```python
from build123d import *

# Parameters (mm, degrees)
MODEL_R                 = 6
MODEL_W                 = 24
MODEL_H                 = 3
SALIENTE_EXTRUIR1_DEPTH = 3


with BuildPart() as part:
    # Model → Saliente-Extruir1 (new body)
    with BuildSketch(Plane.XY):
        Polygon((11.392528896, 93.193403392), (11.392528896, 86.093403392), (23.192528896, 86.093403392), (23.192528896, 62.893403392), (11.392528896, 62.893403392), (11.392528896, 57.193403392), (14.392528896, 57.193403392), (14.392528896, 54.193403392), (11.392528896, 54.193403392), (11.392528896, 51.393403392), (29.392528896, 51.393403392), (29.392528896, 24.993403392), (11.392528896, 24.993403392), (11.392528896, 22.193403392), (14.392528896, 22.193403392), (14.392528896, 19.193403392), (11.392528896, 19.193403392), (11.392528896, -64.806596608), (109.392528896, -64.806596608), (109.392528896, 19.193403392), (106.392528896, 19.193403392), (106.392528896, 22.193403392), (109.392528896, 22.193403392), (109.392528896, 24.993403392), (91.392528896, 24.993403392), (91.392528896, 51.393403392), (109.392528896, 51.393403392), (109.392528896, 54.193403392), (106.392528896, 54.193403392), (106.392528896, 57.193403392), (109.392528896, 57.193403392), (109.392528896, 62.893403392), (97.592528896, 62.893403392), (97.592528896, 86.093403392), (109.392528896, 86.093403392), (109.392528896, 93.193403392), align=None)
        with Locations((60.291833129, 65.722966384)):
            Circle(MODEL_R, mode=Mode.SUBTRACT)
        with Locations((60.392528896, 84.693403392)):
            Rectangle(MODEL_W, MODEL_H, mode=Mode.SUBTRACT)
    extrude(amount=SALIENTE_EXTRUIR1_DEPTH)


solid = part.part
```
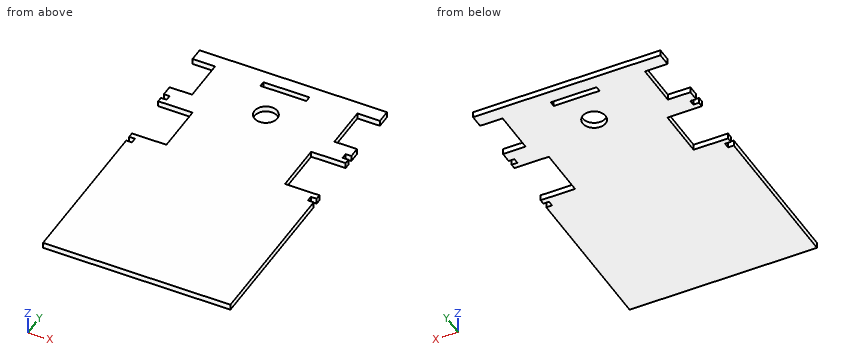
Model file for the job. Use its own axes, mm. Give positions to 0.01 mm unless a question says otherwise; leave off trailing zeros. Write each loop counter-clockwise with the first axis right and the second up, starting at its lowest first coordinate (ties: lowest second). Pieces come first, ordered by that corner, then holes. Notation, with made-up numbers: M -7,-13.75 L 28,-13.75 A18 ccw 28,4.25 Z; hole C 32.5,-28 d9. An arc over 180 degrees is marked long. Use a Markdown table: item, result.
1) Drill centre lines: line 1 (Y direction, x = 101.5, z = 1.05); line 2 (Y direction, x = 94.5, z = 2.3); line 3 (Y direction, x = 56, z = 2.8). Where is each one in solid material? Low to high. Write a range as from..to.
Responses:
| item | result |
|---|---|
| line 1 | y = -64.81..24.99, 51.39..62.89, 86.09..93.19 |
| line 2 | y = -64.81..24.99, 51.39..93.19 |
| line 3 | y = -64.81..61.53, 69.92..83.19, 86.19..93.19 |
2) Cut at C-C (z = 1.2). Give the number of separate pieces and of enclosed holes in the cut face, and give its area (3 significant figures).
Responses:
| item | result |
|---|---|
| separate pieces | 1 |
| enclosed holes | 2 |
| area | 13,800 mm2 |
3) Cut at A-A (x = 102). List the corners of the cut face in (y, z), and give its area (3 significant figures).
Responses:
| item | result |
|---|---|
| outline | M -64.81,0 L 24.99,0 L 24.99,3 L -64.81,3 Z; M 51.39,0 L 62.89,0 L 62.89,3 L 51.39,3 Z; M 86.09,0 L 93.19,0 L 93.19,3 L 86.09,3 Z |
| area | 325 mm2 |
4) Cut at B-B (x = 70.5). List the corners of the cut face in (y, z), and give its area (3 significant figures).
Responses:
| item | result |
|---|---|
| outline | M -64.81,0 L 83.19,0 L 83.19,3 L -64.81,3 Z; M 86.19,0 L 93.19,0 L 93.19,3 L 86.19,3 Z |
| area | 465 mm2 |
5) Pin check, flat tip, straight feed: pin 1 (1.5 mm diameter, centred on y = 56, z = 2, fed in from +X). Stop position of the tip, or through.
Responses:
| item | result |
|---|---|
| pin 1 | stops at x = 106.39 |
